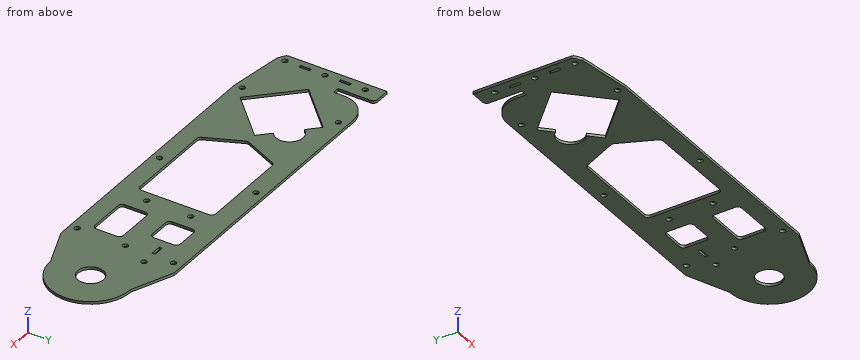
```python
from build123d import *

# Parameters (mm, degrees)
SKETCH_1_R      = 2.05
SKETCH_1_W      = 2.1
SKETCH_1_H      = 8.1
SKETCH_1_R_2    = 2
SKETCH_1_R_3    = 9.525
SKETCH_1_W_2    = 21.362756018
SKETCH_1_H_2    = 20.918096029
SKETCH_1_W_3    = 8.2
SKETCH_1_H_3    = 2.2
EXTRUDE_1_DEPTH = 2
FILLET_1_R      = 3
FILLET_2_R      = 20
FILLET_4_R      = 3


with BuildPart() as part:
    # 草图1 → 凸台-拉伸1 (new body)
    with BuildSketch(Plane.XY):
        with BuildLine():
            Line((240.542857143, -41.815743938), (270.542857143, -30.045714286))
            ThreePointArc((270.542857143, -30.045714286), (300.442857143, -0.145714286), (270.542857143, 29.754285714))
            Line((270.542857143, 29.754285714), (239.574018739, 42.359033922))
            Line((239.574018739, 42.359033922), (13.642857143, 42.359033922))
            Line((13.642857143, 42.359033922), (13.642857143, 14.854285714))
            Line((13.642857143, 14.854285714), (8.642857143, 14.854285714))
            Line((8.642857143, 14.854285714), (8.642857143, 42.359033922))
            Line((8.642857143, 42.359033922), (-5.357142857, 42.359033922))
            Line((-5.357142857, 42.359033922), (-5.357142857, -32.689201643))
            Line((-5.357142857, -32.689201643), (0.542857143, -36.145714286))
            Line((0.542857143, -36.145714286), (40.542857143, -41.815743938))
            Line((40.542857143, -41.815743938), (240.542857143, -41.815743938))
        make_face()
        with Locations((40.542857143, -36.145714286)):
            Circle(SKETCH_1_R, mode=Mode.SUBTRACT)
        with Locations((0.542857143, -30.145714286)):
            Circle(SKETCH_1_R, mode=Mode.SUBTRACT)
        with Locations((135.542857143, -36.145714286)):
            Circle(SKETCH_1_R, mode=Mode.SUBTRACT)
        with Locations((0.542857143, -15.145714286)):
            Rectangle(SKETCH_1_W, SKETCH_1_H, mode=Mode.SUBTRACT)
        with Locations((0.542857143, -0.145714286)):
            Circle(SKETCH_1_R, mode=Mode.SUBTRACT)
        with BuildLine():
            Line((50.542857143, 30.966984086), (59.099206329, 22.4106349))
            ThreePointArc((59.099206329, 22.4106349), (74.584487703, 23.895916275), (73.099206329, 8.4106349))
            Line((73.099206329, 8.4106349), (81.655555515, -0.145714286))
            Line((81.655555515, -0.145714286), (50.542857143, -31.258412658))
            Line((50.542857143, -31.258412658), (19.430158771, -0.145714286))
            Line((19.430158771, -0.145714286), (50.542857143, 30.966984086))
        make_face(mode=Mode.SUBTRACT)
        Polygon((102.300999077, -28.676695157), (89.464558906, -0.145714286), (102.300999077, 27.804285714), (172.548041202, 27.804285714), (172.548041202, -28.676695157), align=None, mode=Mode.SUBTRACT)
        with Locations((230.542857143, -36.145714286)):
            Circle(SKETCH_1_R, mode=Mode.SUBTRACT)
        with Locations((180.542857143, -16.645714286)):
            Circle(SKETCH_1_R_2, mode=Mode.SUBTRACT)
        Polygon((224.574018739, -28.676695157), (213.241022587, -28.676695157), (191.878266569, -28.676695157), (191.878266569, -7.415485794), (224.574018739, -7.415485794), align=None, mode=Mode.SUBTRACT)
        with Locations((230.542857143, -0.145714286)):
            Circle(SKETCH_1_R_2, mode=Mode.SUBTRACT)
        with Locations((270.542857143, -0.145714286)):
            Circle(SKETCH_1_R_3, mode=Mode.SUBTRACT)
        with Locations((0.542857143, 14.854285714)):
            Rectangle(SKETCH_1_W, SKETCH_1_H, mode=Mode.SUBTRACT)
        with Locations((0.542857143, 29.854285714)):
            Circle(SKETCH_1_R, mode=Mode.SUBTRACT)
        with Locations((40.542857143, 35.854285714)):
            Circle(SKETCH_1_R, mode=Mode.SUBTRACT)
        with Locations((135.542857143, 35.854285714)):
            Circle(SKETCH_1_R, mode=Mode.SUBTRACT)
        with Locations((180.542857143, 16.354285714)):
            Circle(SKETCH_1_R_2, mode=Mode.SUBTRACT)
        with Locations((202.559644578, 17.3452377)):
            Rectangle(SKETCH_1_W_2, SKETCH_1_H_2, mode=Mode.SUBTRACT)
        with Locations((224.574018739, 19.704285714)):
            Rectangle(SKETCH_1_W_3, SKETCH_1_H_3, mode=Mode.SUBTRACT)
        with Locations((239.574018739, 19.704285714)):
            Circle(SKETCH_1_R, mode=Mode.SUBTRACT)
        with Locations((230.542857143, 35.854285714)):
            Circle(SKETCH_1_R, mode=Mode.SUBTRACT)
    extrude(amount=EXTRUDE_1_DEPTH)

    # 圆角1
    fillet_1_edges = [part.edges().sort_by_distance(p)[0] for p in [
        (224.574018739, -7.415485794, 1),
        (191.878266569, -7.415485794, 1),
        (191.878266569, -28.676695157, 1),
        (224.574018739, -28.676695157, 1),
        (172.548041202, -28.676695157, 1),
        (172.548041202, 27.804285714, 1),
        (102.300999077, 27.804285714, 1),
        (89.464558906, -0.145714286, 1),
        (102.300999077, -28.676695157, 1),
        (191.878266569, 27.804285714, 1),
        (191.878266569, 6.886189685, 1),
        (213.241022587, 6.886189685, 1),
        (213.241022587, 27.804285714, 1),
    ]]
    fillet(fillet_1_edges, radius=FILLET_1_R)

    # 圆角2
    fillet_2_edges = [part.edges().sort_by_distance(p)[0] for p in [
        (13.642857143, 42.359033922, 1),
    ]]
    fillet(fillet_2_edges, radius=FILLET_2_R)

    # 圆角4
    fillet_4_edges = [part.edges().sort_by_distance(p)[0] for p in [
        (40.542857143, -41.815743938, 1),
        (0.542857143, -36.145714286, 1),
        (-5.357142857, -32.689201643, 1),
        (8.642857143, 42.359033922, 1),
    ]]
    fillet(fillet_4_edges, radius=FILLET_4_R)


solid = part.part
```
Build history of the part. All positions in model axes, mm. Round coordinates to 2 decimals unless told otherwise and drop trailing zeros. Write each loop counter-clockwise with the first axis right and the second up, starting at its lowest first coordinate (ties: lowest second). Pieces come first, ordered by that corner, then holes. Notation, with made-up numbers: (67, -26.5) -> (119, -26.5) arc R21 cw to (119, -10.5) -> close; hole circle Ø7 at (82.25, 39). An arc over 180 degrees is marked (long way). Put each result on its own line as item: value.
Item 1: Wall check: probe 1 along Y at (x, z) = (128.5, 1.8); probe 2 along X at (y, z) = (21.5, 1.95); probe 3 along X at (y, z) = (-6, 1.2). Give the ranges that are in metal, low to high. Write a range as from..to.
Here are the results:
probe 1: y = -41.82..-28.68, 27.8..42.36
probe 2: x = -5.36..8.64, 13.64..41.08, 76.36..99.41, 172.55..191.88, 213.24..238.59, 240.56..291.17
probe 3: x = -5.36..25.28, 75.8..92.1, 172.55..263.03, 278.06..299.86
Item 2: Slice it at C-C, the plane x = 46. Give the cut face in (y, z).
Here are the results:
outline: (-41.82, 0) -> (-26.72, 0) -> (-26.72, 2) -> (-41.82, 2) -> close; (26.42, 0) -> (42.36, 0) -> (42.36, 2) -> (26.42, 2) -> close
Item 3: Flat gauge pins, fed straight in: P1, Ø12, axis at x = 67.45, y = 16.77, coming from the +Z side; P2, Ø0.6, axis at y = -21, z = 1, coming from the +X side; P3, Ø0.6, axis at x = 10.5, z = 1, coming from the +Y side; P4, Ø1, axis at y = 32, z = 1, coming from the +X side. Where does each tip first touch, or does it go through?
Here are the results:
P1: passes through
P2: stops at x = 292.26
P3: stops at y = 14.85
P4: stops at x = 266.25
Item 4: Slice it at A-A, the plane x = 108. Give the cut face in (y, z).
Here are the results:
outline: (-41.82, 0) -> (-28.68, 0) -> (-28.68, 2) -> (-41.82, 2) -> close; (27.8, 0) -> (42.36, 0) -> (42.36, 2) -> (27.8, 2) -> close
Item 5: Slice it at D-D, the plane z = 0.5. Count the separate pieces of the cut face and the enclosed holes in it, plus the area to 3 significant figures.
Here are the results:
separate pieces: 1
enclosed holes: 21
area: 15,800 mm^2
Item 6: Slice it at B-B, the plane x = 202. Give the cut face in (y, z), plus the area to 3 significant figures.
Here are the results:
outline: (-41.82, 0) -> (-28.68, 0) -> (-28.68, 2) -> (-41.82, 2) -> close; (-7.42, 0) -> (6.89, 0) -> (6.89, 2) -> (-7.42, 2) -> close; (27.8, 0) -> (42.36, 0) -> (42.36, 2) -> (27.8, 2) -> close
area: 84.0 mm^2
